Here's the drawing with two shaded views (mm, measured from the low corner). I have some questions. Give positions to 0.01 mm unless a question says otherwise; leave off trailing zeros. Write each loop counter-clockwise with the first axis right and the second up, starting at its lowest first coordinate (ties: lowest second). Pieces come first, ordered by that corner, then holes. Notation, with made-up numbers: (29, 45.5) -> (84, 45.5) arc R9 cw to (84, 57.5) -> close; hole circle Ø6 at (89.25, 26). An arc over 180 degrees is marked (long way). One line per item, written item: value.
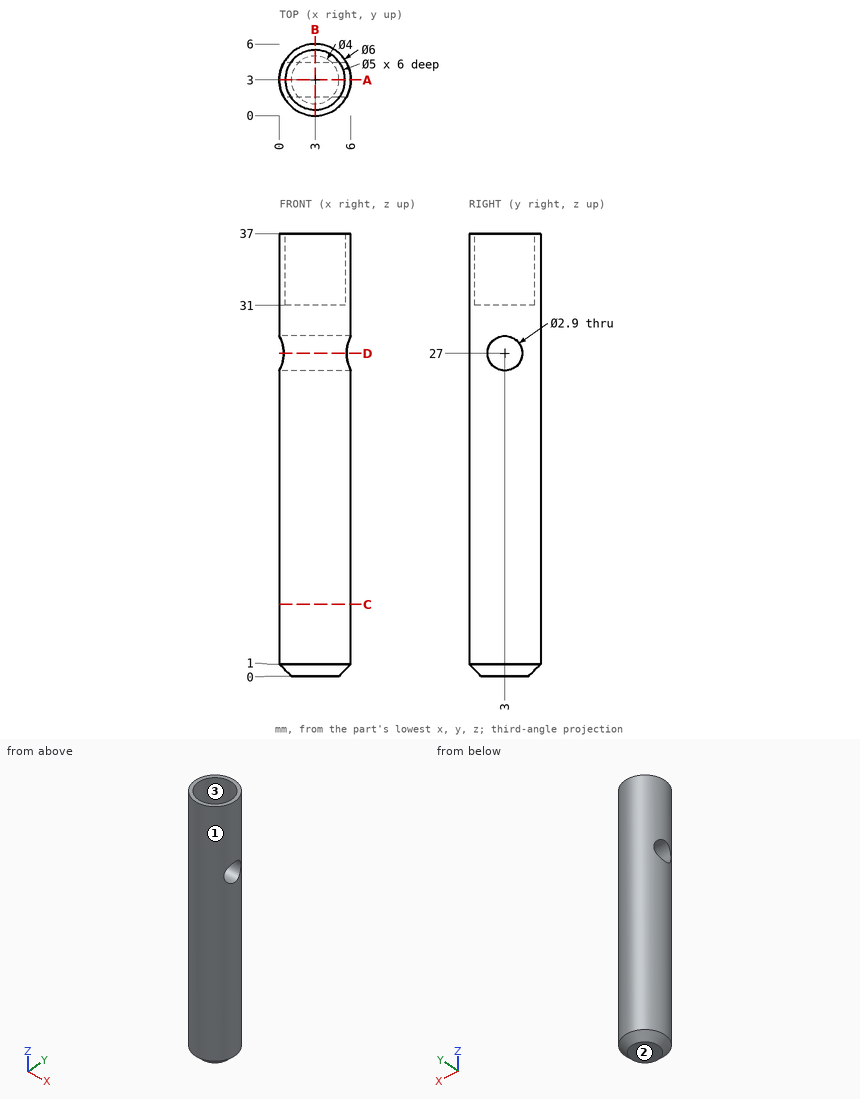
1) Will this pin go through, and if not, where does the flat tip stop? pin 1 (1.5 mm diameter, centred on x = 3, y = 3.5, fed in from +Z).
Answer list:
pin 1: stops at z = 31
2) If we section it at A-A (y = 3): Write out the boundary of the cut face in (x, z), and give its area (3 significant figures).
Answer list:
outline: (0, 1) -> (1, 0) -> (5, 0) -> (6, 1) -> (6, 25.55) -> (0, 25.55) -> close; (0, 28.45) -> (6, 28.45) -> (6, 37) -> (5.5, 37) -> (5.5, 31) -> (0.5, 31) -> (0.5, 37) -> (0, 37) -> close
area: 174 mm^2
3) If we section it at D-D (z = 27): Write out the boundary of the cut face in (x, y), and give its area (3 significant figures).
Answer list:
outline: (0.37, 1.55) arc R3 ccw to (5.63, 1.55) -> close; (0.37, 4.45) -> (5.63, 4.45) arc R3 ccw to start
area: 11.6 mm^2
4) If we section it at B-B (x = 3): Write out the boundary of the cut face in (y, z).
Answer list:
outline: (0, 1) -> (1, 0) -> (5, 0) -> (6, 1) -> (6, 37) -> (5.5, 37) -> (5.5, 31) -> (0.5, 31) -> (0.5, 37) -> (0, 37) -> close; hole circle Ø2.9 at (3, 27)
5) We'd pull the mould along Y, two halves only. Please class the marked faces 1, 2 and 3: released by +Y, released by -Y, zero draft, split by the parting line, or undercut.
Answer list:
face 1: split by the parting line
face 2: zero draft
face 3: undercut
6) If we section it at C-C (z = 6): Write out the boundary of the cut face in (x, y).
Answer list:
outline: circle Ø6 at (3, 3)
7) I need wall thicknesses on L1, parallel to Y at x = 3, z = 34.9; L2, parallel to Z at x = 1.5, y = 3.75; L3, parallel to Y at x = 3.75, z = 27. Which ranges of each line are inside material? Lowest first, please.
Answer list:
L1: y = 0 to 0.5, 5.5 to 6
L2: z = 0 to 25.76, 28.24 to 31
L3: y = 0.1 to 1.55, 4.45 to 5.9
